The model under review builds one solid part; all positions refer to its coordinate system, in mm. Face numbers are marked on the shaded views. Coordinates: 2 decimals unless noted, no trailing zeros. Loops run counter-clockwise (first coordinate to the right, second up) from the corner with the lowest first, then second, coordinate; pieces in that order, holes last. Notation, with made-up numbers: M -36.75,-38 L 1.25,-38 A14 ccw 1.25,-18 Z; hole C 73.25,-3.5 d11. An arc over 180 degrees is marked long. Return JSON: item names as keys, results as strings.
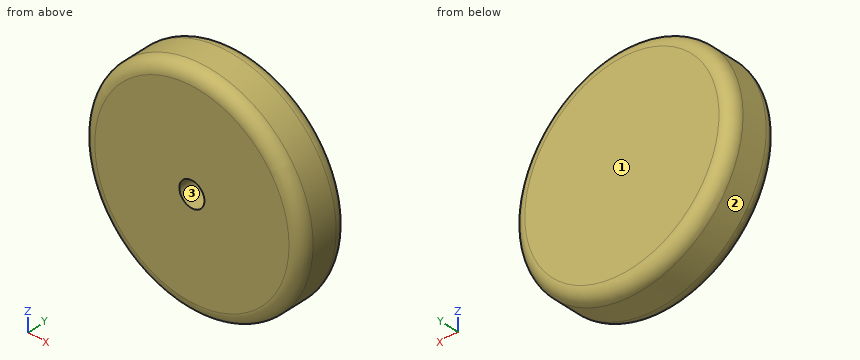
```python
from build123d import *

# Parameters (mm, degrees)
F0_R     = 44.45
F1_DEPTH = 20.32
F2_R     = 5.08
F3_DEPTH = 18.542
F4_R     = 5.08


with BuildPart() as f1:
    # F0 (on Front) → F1 (new body)
    with BuildSketch(Plane.XZ):
        Circle(F0_R)
    extrude(amount=F1_DEPTH)

    # F2 (on face) → F3 (cut)
    with BuildSketch(Plane.XZ.offset(20.32)):
        Circle(F2_R)
    extrude(amount=-F3_DEPTH, mode=Mode.SUBTRACT)

    # F4
    f4_edges = [f1.edges().sort_by_distance(p)[0] for p in [
        (-44.45, -20.32, 0),
        (-44.45, 0, 0),
    ]]
    fillet(f4_edges, radius=F4_R)


solid = f1.part
```
1. To check wall thickness, follow line 1 (Z direction, x = 0, y = -5.25); line 2 (Z direction, x = 0, y = -16.25); line 3 (X direction, y = -14.5, z = 37). State the ranges of each line that lie inside material, in increasing order.
Check values:
{"line 1": "-44.45 to -5.08, 5.08 to 44.45", "line 2": "-44.35 to -5.08, 5.08 to 44.35", "line 3": "-24.63 to 24.63"}
2. Add section B-B on z = 0. Give the boundary of the cut face in (x, y), plus the area to 3 significant figures.
Check values:
{"outline": "M -44.45,-15.24 A5.08 ccw -39.37,-20.32 L -5.08,-20.32 L -5.08,-1.78 L 5.08,-1.78 L 5.08,-20.32 L 39.37,-20.32 A5.08 ccw 44.45,-15.24 L 44.45,-5.08 A5.08 ccw 39.37,0 L -39.37,0 A5.08 ccw -44.45,-5.08 Z", "area": "1,600 mm²"}
3. Add section D-D on y = -17. Give the boundary of the cut face in (x, z), plus the area to 3 significant figures.
Check values:
{"outline": "C 0,0 d88.27; hole C 0,0 d10.16", "area": "6,040 mm²"}
4. Add section A-A on x = 0. Give the boundary of the cut face in (y, z).
Check values:
{"outline": "M -20.32,-39.37 A5.08 ccw -15.24,-44.45 L -5.08,-44.45 A5.08 ccw 0,-39.37 L 0,39.37 A5.08 ccw -5.08,44.45 L -15.24,44.45 A5.08 ccw -20.32,39.37 L -20.32,5.08 L -1.78,5.08 L -1.78,-5.08 L -20.32,-5.08 Z"}
5. The part is to be moulded in two halves that separate along Z. For the marked faces 1, 2 and 3, say which applies: released by +Z, released by -Z, zero draft, split by the parting line, or undercut.
Check values:
{"face 1": "zero draft", "face 2": "split by the parting line", "face 3": "undercut"}
6. Add section C-C on y = -6.5. Give the boundary of the cut face in (x, z), plus the area to 3 significant figures.
Check values:
{"outline": "C 0,0 d88.9; hole C 0,0 d10.16", "area": "6,130 mm²"}
7. Insertion check: pin 1 Ø1 at (x, y) = (5.5, -13.5) entering from -Z; pin 2 Ø12 at (y, z) = (-16, -35) entering from +X; pin 3 Ø4 at (x, y) = (-13.5, -14) entering from -Z. Each pin has a flat end and moves straight along its axis. Give the tip position at first contact, or say it passes through.
Check values:
{"pin 1": "z = -44.17", "pin 2": "x = 33.66", "pin 3": "z = -42.94"}
